Here's how the part is built. I have some questions about the finished solid (model axes, mm). Face numbers are marked on the shaded views. A direction names the side the tool comes from. Coordinates: 2 decimals unless noted, no trailing zeros. Write each loop counter-clockwise with the first axis right and the second up, starting at its lowest first coordinate (ties: lowest second). Pieces come first, ordered by that corner, then holes.
(1) Please list where these lines run through material, in increasing order: probe 1 along Z at (x, y) = (-10, 11.35); probe 2 along Y at (x, z) = (0, 0.75); probe 3 along Y at (x, z) = (-8, 1).
(2) Imagine slicing it at A-A, the plane y = 10. List the corners of the cut face in (x, z) for me, plus the area to 3 significant figures.
(3) Imagine slicing it at B-B, the plane z = 7. List the corners of the cut face in (x, y) for me, plus the area to 3 significant figures.
(4) Imagine slicing it at D-D, the plane y = -10. List the corners of the cut face in (x, z) for me.
(5) Thinking about a two-plate mould opening in X: for the marked faces 1, 2 and 3, which applies, released by +X, released by -X, zero draft, split by the parting line, or undercut?
(6) Imagine slicing it at C-C, the plane x = 0. List the corners of the cut face in (y, z) for me.
(7) For pin 1 Ø2.5 at (x, z) = (-10, 4) entering from -Y; pin 2 Ø2.5 at (x, y) = (12.12, -7) entering from -Z; pin 3 Ø2 at (x, z) = (-1, 4) entering from -Y; pin 4 Ø2 at (x, z) = (-10.5, 3) entering from -Y, each with a flat end and sliding along its axis, tell me the tip position at first contact or that it passes through.
(8) Which directions (+Z, -Z, +X, -X, +Y, -Y) give clear straight access to the entire face, cutting with the end or side of a thin tool? Please do the marked faces 4 and 5.
```python
from build123d import *

# Parameters (mm, degrees)
SKETCH1_R           = 1.5
SKETCH1_R_2         = 11
BOSS_EXTRUDE1_DEPTH = 8
SKETCH4_W           = 7.1
SKETCH4_H           = 3.2
CUT_EXTRUDE1_DEPTH  = 32.148836254
SKETCH5_R           = 2.05
CUT_EXTRUDE2_DEPTH  = 14


with BuildPart() as part:
    # Sketch1 → Boss-Extrude1 (new body)
    with BuildSketch(Plane.XY):
        with BuildLine():
            Line((-19, 0), (-20, 22.5))
            Line((-20, 22.5), (20, 22.5))
            Line((20, 22.5), (19, 0))
            ThreePointArc((19, 0), (0, -19), (-19, 0))
        make_face()
        with Locations((0, 14)):
            Circle(SKETCH1_R, mode=Mode.SUBTRACT)
        Circle(SKETCH1_R_2, mode=Mode.SUBTRACT)
        with Locations((12.124355653, -7)):
            Circle(SKETCH1_R, mode=Mode.SUBTRACT)
        with Locations((-12.124355653, -7)):
            Circle(SKETCH1_R, mode=Mode.SUBTRACT)
    extrude(amount=BOSS_EXTRUDE1_DEPTH)

    # Sketch4 → Cut-Extrude1 (cut, through all)
    with BuildSketch(Plane.XY.offset(8)):
        with Locations((-10, 13.9)):
            Rectangle(SKETCH4_W, SKETCH4_H)
        with Locations((10, 13.9)):
            Rectangle(SKETCH4_W, SKETCH4_H)
    extrude(amount=-CUT_EXTRUDE1_DEPTH, mode=Mode.SUBTRACT)

    # Sketch5 → Cut-Extrude2 (cut)
    with BuildSketch(Plane(origin=(0, 22.5, 0), x_dir=(1, 0, 0), z_dir=(0, 1, 0))):
        with Locations(Location((-10, -4, 0), (0, 0, 180))):
            Circle(SKETCH5_R)
        with Locations(Location((10, -4, 0), (0, 0, 180))):
            Circle(SKETCH5_R)
    extrude(amount=-CUT_EXTRUDE2_DEPTH, mode=Mode.SUBTRACT)


solid = part.part
```
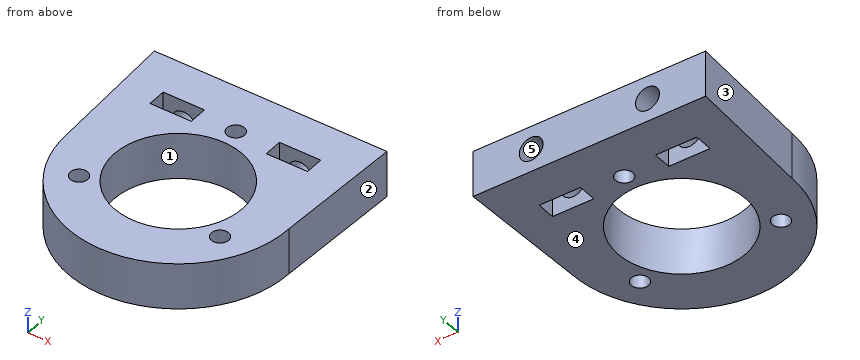
Recorded:
1. probe 1: z = 0 to 1.95, 6.05 to 8
1. probe 2: y = -19 to -11, 11 to 12.5, 15.5 to 22.5
1. probe 3: y = -17.23 to -7.55, 7.55 to 12.3, 15.5 to 22.5
2. outline: (-19.44, 0) - (-4.58, 0) - (-4.58, 8) - (-19.44, 8) - close; (4.58, 0) - (19.44, 0) - (19.44, 8) - (4.58, 8) - close; hole circle Ø4.1 at (-10, 4); hole circle Ø4.1 at (10, 4)
2. area: 211 mm2
3. outline: (-20, 22.5) - (-19, 0) arc R19 ccw to (19, 0) - (20, 22.5) - close; hole circle Ø3 at (-12.12, -7); hole (-13.55, 12.3) - (-6.45, 12.3) - (-6.45, 15.5) - (-13.55, 15.5) - close; hole circle Ø22 at (0, 0); hole circle Ø3 at (0, 14); hole (6.45, 12.3) - (13.55, 12.3) - (13.55, 15.5) - (6.45, 15.5) - close; hole circle Ø3 at (12.12, -7)
3. area: 998 mm2
4. outline: (-16.16, 0) - (-4.58, 0) - (-4.58, 8) - (-16.16, 8) - close; (4.58, 0) - (16.16, 0) - (16.16, 8) - (4.58, 8) - close
5. face 1: undercut
5. face 2: released by +X
5. face 3: released by -X
6. outline: (-19, 0) - (-11, 0) - (-11, 8) - (-19, 8) - close; (11, 0) - (12.5, 0) - (12.5, 8) - (11, 8) - close; (15.5, 0) - (22.5, 0) - (22.5, 8) - (15.5, 8) - close
7. pin 1: stops at y = -16.87
7. pin 2: passes through
7. pin 3: stops at y = -19
7. pin 4: stops at y = -16.45
8. face 4: -Z, +X, -X, +Y, -Y
8. face 5: +Y
